from build123d import *


with BuildPart() as part:
    # Sketch2 → Revolve1 (revolve)
    with BuildSketch(Plane(origin=(0, 0, 0), x_dir=(1, 0, 0), z_dir=(0, 1, 0))):
        with BuildLine():
            Line((0, 0), (0, 13))
            Line((0, 13), (0.8, 13))
            Line((0.8, 13), (0.8, 9.417496864))
            ThreePointArc((0.8, 9.417496864), (0.851837315, 9.013526198), (1.003990374, 8.635731474))
            Line((1.003990374, 8.635731474), (3.141788619, 4.81823461))
            ThreePointArc((3.141788619, 4.81823461), (3.728732309, 4.219633269), (4.537798244, 4))
            Line((4.537798244, 4), (5.168545919, 4))
            ThreePointArc((5.168545919, 4), (5.414855468, 4.128735275), (5.449773501, 4.404455959))
            Line((5.449773501, 4.404455959), (3, 11))
            Line((3, 11), (3.8, 11))
            Line((3.8, 11), (6.012636566, 5.042901553))
            ThreePointArc((6.012636566, 5.042901553), (6.599105133, 4.286349073), (7.512517001, 4))
            Line((7.512517001, 4), (7.568545919, 4))
            ThreePointArc((7.568545919, 4), (7.814855468, 4.128735275), (7.849773501, 4.404455959))
            Line((7.849773501, 4.404455959), (5.4, 11))
            Line((5.4, 11), (6.2, 11))
            Line((6.2, 11), (8.699880435, 4.269552674))
            ThreePointArc((8.699880435, 4.269552674), (8.774771205, 3.995465979), (8.8, 3.712454227))
            Line((8.8, 3.712454227), (8.8, 0))
            Line((8.8, 0), (0, 0))
        make_face()
    revolve(axis=Axis((8.8, 0, 0), (-1, 0, 0)))


solid = part.part
Part model, mm, in its own coordinate system. A direction names the side the tool comes from. Coordinates: 2 decimals unless noted, no trailing zeros. Loops run counter-clockwise (first coordinate to the right, second up) from the corner with the lowest first, then second, coordinate; pieces in that order, holes last. Notation, with made-up numbers: M -23,88 L 0,88 A24 cw 0,104 Z; hole C 18.25,-20 d10. An arc over 180 degrees is marked long. Use a Markdown table: item, result. Add a question column.
Q1. Probe L1, parallel to X at y = 6.25, z = -6.5; L2, parallel to X at y = 6.5, z = 1.5; L3, parallel to X at y = -7.25, z = 9.5. List the from-to ranges inside material, lowest first.
Q2. Mould opens along X. For faces 1 (the cylindrical face through (5.81, 10.74, 2.38)), 2 (the flat face through (8.8, 0, 0)), 3 (the flat face through (0.8, -4, -9)) say: +X half, -X half, draft (parallel to the pull), parting line (faces both ways), or undercut.
Q3. Cut at B-B (x = 2.5). Write the cut outline in (y, z).
Q4. Cut at A-A (x = 7). Write the cut outline in (y, z), and give its area (3 significant figures).
Q5. Which spindle directions (+Z, -Z, +X, -X, +Y, -Y) get a long thin tool onto all of the face, cutting with end or side? Do faces 4 (the conical face through (3.04, -4.96, 0.65)), 5 (the cylindrical face through (0.406, 7.91, 10.316)), 6 (the cylindrical face through (3.41, 10.74, 2.38)). Say none if no direction does.
Q6. Pin check, flat tips, straight feed: P1, Ø5, axis at x = 5, y = -6.5, coming from the -Z side; P2, Ø5, axis at y = 7, z = 2, coming from the +X side; P3, Ø1.5, axis at x = 2.5, z = 2, coming from the +Y side. Stop position of each tip, or through.
Worked out:
| question | item | result |
|---|---|---|
| 1 | L1 | x = 0 to 0.85, 3.74 to 4.54, 6.14 to 6.94 |
| 1 | L2 | x = 0 to 2.1, 4.61 to 5.41, 7.01 to 7.81 |
| 1 | L3 | x = 0 to 0.8 |
| 2 | face 1 | draft |
| 2 | face 2 | +X half |
| 2 | face 3 | undercut |
| 3 | outline | C 0,0 d11.93 |
| 4 | outline | C 0,0 d17.69; C 0,0 d8.17; hole C 0,0 d13.38 |
| 4 | area | 158 mm2 |
| 5 | face 4 | none |
| 5 | face 5 | +X, -X |
| 5 | face 6 | +X |
| 6 | P1 | stops at z = -10.23 |
| 6 | P2 | stops at x = 8.51 |
| 6 | P3 | stops at y = 10.91 |
